```python
from build123d import *

# Parameters (mm, degrees)
SKETCH_1_R      = 1
EXTRUDE_1_DEPTH = 12.5
EXTRUDE_2_DEPTH = 1
EXTRUDE_3_REACH = 18.039
SKETCH_3_W      = 5
SKETCH_3_H      = 1
FILLET_1_R      = 1


with BuildPart() as part:
    # Sketch 1 → Extrude 1 (new body)
    with BuildSketch(Plane.XY):
        Circle(SKETCH_1_R)
    extrude(amount=EXTRUDE_1_DEPTH)

    # Sketch 3 → Extrude 3 (add, up to next)
    with BuildSketch(Plane.ZY.offset(-1), mode=Mode.PRIVATE) as extrude_3_sk1:
        with Locations((8, -0.5)):
            Rectangle(SKETCH_3_W, SKETCH_3_H)
    extrude_3_tool1 = extrude(extrude_3_sk1.sketch, amount=EXTRUDE_3_REACH, mode=Mode.PRIVATE) - part.part


with BuildPart() as body_2:
    # Sketch 2 → Extrude 2 (new body)
    with BuildSketch(Plane(origin=(0, 0, 0), x_dir=(1, 0, 0), z_dir=(0, 1, 0))):
        Polygon((1, -10.5), (1, -5.5), (11, -4.625113365), (11, -11.374886635), align=None)
    extrude(amount=-EXTRUDE_2_DEPTH)


with BuildPart() as part_1:
    add(part.part)

    add(body_2.part)  # Extrude 3 merges body 2
    add(extrude_3_tool1.solids().sort_by_distance((1, -0.5, 8))[0])

    # Sketch 5 → Revolve 2 (revolve)
    with BuildSketch(Plane(origin=(0, 0, 0), x_dir=(1, 0, 0), z_dir=(0, 1, 0)), mode=Mode.PRIVATE) as revolve_2_sk:
        Polygon((-1, -12.5), (-0.35, -14.2), (-0.35, -38.2), (0, -38.2), (0, -14.2), (0, -12.5), align=None)
    revolve(revolve_2_sk.sketch.rotate(Axis((0, 0, 38.2), (0, 0, -1)), 180), axis=Axis((0, 0, 38.2), (0, 0, -1)))

    # Fillet 1
    fillet_1_edges = [part_1.edges().sort_by_distance(p)[0] for p in [
        (11, -0.5, 11.374886635),
        (11, -0.5, 4.625113365),
    ]]
    fillet(fillet_1_edges, radius=FILLET_1_R)


solid = part_1.part
```
For this review, take the finished solid that the model builds, in its own axes (mm). A direction names the side the tool comes from. Round coordinates to 2 decimals unless told otherwise and drop trailing zeros. Write each loop counter-clockwise with the first axis right and the second up, starting at its lowest first coordinate (ties: lowest second). Pieces come first, ordered by that corner, then holes. Notation, with made-up numbers: (64.25, 78.5) -> (109.25, 78.5) arc R14 cw to (109.25, 84.5) -> close; hole circle Ø6 at (87, 53.25). An arc over 180 degrees is marked (long way). Use one line per item in the form item = value.
Q1. Consider section A-A (z = 2). State the section outline as (x, y) points.
Resolved:
outline = circle Ø2 at (0, 0)
Q2. Machinability: for faces 1 (the flat face through (5.394, -0.493, 5.116)), 2 (the flat face through (11, -0.5, 8)), which of the approach directions +Z, -Z, +X, -X, +Y, -Y give a long, thin tool a straight path to every point of the face, cutting with its end or side? Answer none if there is none.
Resolved:
face_1 = -Z, +Y, -Y
face_2 = +Z, -Z, +X, +Y, -Y
Q3. The part is to be moulded in two halves that separate along X. For faces 3 (the flat face through (5.519, -0.493, 10.895)), 4 (the flat face through (6, 0, 8)), 5 (the conical face through (-0.13, 0.584, 13.551)), say which applies: released by +X, released by -X, zero draft, split by the parting line, or undercut.
Resolved:
face_3 = undercut
face_4 = zero draft
face_5 = split by the parting line
Q4. Clearance check with a flat-ended pin moving along its axis: pin 1 Ø5.5 at (x, z) = (6.5, 6.5) entering from +Y. State where the tip first meets the part, or that it passes through.
Resolved:
pin_1 = 0
Q5. Consider section C-C (z = 8). State the section outline as (x, y) points, then the cut area to 3 significant figures.
Resolved:
outline = (0, -1) -> (11, -1) -> (11, 0) -> (1, 0) arc R1 ccw (long way) to start
area = 13.4 mm²
Q6. Consider section D-D (z = 16.5). State the section outline as (x, y) points.
Resolved:
outline = circle Ø0.7 at (0, 0)
Q7. To check wall thickness, follow probe 1 along X at (y, z) = (0.1, 9.5); probe 2 along X at (y, z) = (-0.05, 7.5); probe 3 along Y at (x, z) = (-0.25, 23.5). State the ranges of each line that lie inside material, in increasing order. Write a range as from..to.
Resolved:
probe_1 = -0.99..0.99
probe_2 = -1..11
probe_3 = -0.24..0.24
Q8. Consider section B-B (x = 7). State the section outline as (y, z) points, then the cut area to 3 significant figures.
Resolved:
outline = (-1, 4.98) -> (0, 4.98) -> (0, 11.02) -> (-1, 11.02) -> close
area = 6.05 mm²
